from build123d import *

# Parameters (mm, degrees)
EXTRUDE_1_DEPTH     = 158
SKETCH_2_R          = 1.6
CUT_EXTRUDE_1_DEPTH = 27
SKETCH_6_R          = 3.5
CUT_EXTRUDE_2_DEPTH = 21
SKETCH_7_R          = 2.2
CUT_EXTRUDE_3_DEPTH = 5
CUT_EXTRUDE_4_DEPTH = 10
CUT_EXTRUDE_5_DEPTH = 4


with BuildPart() as part:
    # 草图1 → 凸台-拉伸1 (new body)
    with BuildSketch(Plane.XY):
        Polygon((-43.805178849, 53.227759989), (-48.805178849, 53.227759989), (-70.018382284, 32.014556553), (-67.189955159, 29.186129428), (-48.805178849, 47.570905739), (-48.805178849, 37.570905739), (-43.805178849, 37.570905739), align=None)
    extrude(amount=EXTRUDE_1_DEPTH)

    # 草图2 → 切除-拉伸1 (cut)
    with BuildSketch(Plane(origin=(-43.805178849, 0, 0), x_dir=(0, 0, -1), z_dir=(1, 0, 0))):
        with Locations((-130, 42.570905739)):
            Circle(SKETCH_2_R)
        with Locations((-28, 42.570905739)):
            Circle(SKETCH_2_R)
    extrude(amount=-CUT_EXTRUDE_1_DEPTH, mode=Mode.SUBTRACT)

    # 草图6 → 切除-拉伸2 (cut)
    with BuildSketch(Plane.ZY.offset(48.805178849)):
        with Locations(Location((130, 42.570905739, 0), (0, 0, 90))):
            Circle(SKETCH_6_R)
        with Locations(Location((28, 42.570905739, 0), (0, 0, 90))):
            Circle(SKETCH_6_R)
    extrude(amount=CUT_EXTRUDE_2_DEPTH, mode=Mode.SUBTRACT)

    # 草图7 → 切除-拉伸3 (cut)
    with BuildSketch(Plane(origin=(-51.016469419, 51.016469419, 0), x_dir=(0.7071067811865521, 0.707106781186543, 0), z_dir=(-0.707106781186543, 0.7071067811865521, 0))):
        with Locations(Location((-11.872762886, -148, 0), (0, 0, 180))):
            Circle(SKETCH_7_R)
        with Locations(Location((-11.872762886, -10, 0), (0, 0, 180))):
            Circle(SKETCH_7_R)
    extrude(amount=-CUT_EXTRUDE_3_DEPTH, mode=Mode.SUBTRACT)

    # 草图8 → 切除-拉伸4 (cut)
    with BuildSketch(Plane(origin=(-43.805178849, 0, 0), x_dir=(0, 0, -1), z_dir=(1, 0, 0))):
        Polygon((-158, 53.227759989), (-158, 51.727759989), (-156.5, 53.227759989), align=None)
        Polygon((0, 53.227759989), (-1.5, 53.227759989), (0, 51.727759989), align=None)
        Polygon((-158, 39.070905739), (-158, 37.570905739), (-156.5, 37.570905739), align=None)
        Polygon((0, 37.570905739), (0, 39.070905739), (-1.5, 37.570905739), align=None)
    extrude(amount=-CUT_EXTRUDE_4_DEPTH, mode=Mode.SUBTRACT)

    # 草图9 → 切除-拉伸5 (cut)
    with BuildSketch(Plane(origin=(-48.188042294, 48.188042294, 0), x_dir=(0, 0, -1), z_dir=(0.7071067811865477, -0.7071067811865474, 0))):
        Polygon((-158, -26.872762886), (-158, -25.372762886), (-156.5, -26.872762886), align=None)
        Polygon((0, -26.872762886), (0, -25.372762886), (-1.5, -26.872762886), align=None)
    extrude(amount=-CUT_EXTRUDE_5_DEPTH, mode=Mode.SUBTRACT)


solid = part.part
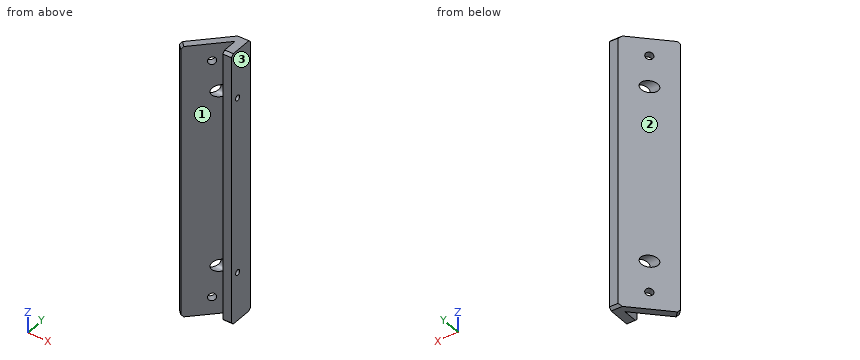
Design review of the part built by this model. Coordinates are the model's own, in mm. Face numbers are marked on the shaded views. Give positions to 0.01 mm unless a question says otherwise; leave off trailing zeros. Write each loop counter-clockwise with the first axis right and the second up, starting at its lowest first coordinate (ties: lowest second). Pieces come first, ordered by that corner, then holes. Notation, with made-up numbers: M -15,47.5 L 42,47.5 A31 ccw 42,72.5 Z; hole C -22.75,63.25 d1. An arc over 180 degrees is marked long. Return JSON: item names as keys, results as strings. Group by question number.
Item 1: Wall thickness on line 1 along Y through (x, z) = (-44.8, 130); line 2 along X through (y, z) = (46.25, 125.5); line 3 along X through (y, z) = (38.25, 87.5): over which ranges is each line inside the solid? List them lowest first.
Item 2: The part is to be moulded in two halves that separate along X. For the marked faces 1, 2 and 3, say which applies: pulls with the +X half, pulls with the -X half, needs draft (parallel to the pull), parting line crosses it, or undercut.
Item 3: Clearance check with flat-ended pins moving along their axes: pin 1 Ø1 at (x, z) = (-65.5, 75) entering from -Y; pin 2 Ø5.5 at (y, z) = (42.57, 28) entering from -X; pin 3 Ø5 at (y, z) = (43, 23) entering from -X. State where each tip first meets the part, or that it passes through.
Item 4: Take a section at B-B (z = 28). Give the boundary of the cut face in (x, y).
Item 5: Take a section at A-A (z = 136). Give the boundary of the cut face in (x, y), plus the area to 3 significant figures.
Return value:
{
 "1": {"line 1": "y = 37.57 to 40.97, 44.17 to 53.23", "line 2": "x = -55.78 to -50.13, -48.81 to -43.81", "line 3": "x = -63.78 to -58.13, -48.81 to -43.81"},
 "2": {"face 1": "undercut", "face 2": "pulls with the -X half", "face 3": "pulls with the +X half"},
 "3": {"pin 1": "stops at y = 30.38", "pin 2": "stops at x = -48.81", "pin 3": "stops at x = -61.53"},
 "4": {"outline": "M -70.02,32.01 L -67.19,29.19 L -57.31,39.07 L -62.96,39.07 Z; M -55.96,46.07 L -50.31,46.07 L -48.81,47.57 L -48.81,44.17 L -43.81,44.17 L -43.81,53.23 L -48.81,53.23 Z; M -48.81,37.57 L -43.81,37.57 L -43.81,40.97 L -48.81,40.97 Z"},
 "5": {"outline": "M -70.02,32.01 L -67.19,29.19 L -48.81,47.57 L -48.81,37.57 L -43.81,37.57 L -43.81,53.23 L -48.81,53.23 Z", "area": "190 mm2"}
}
